from build123d import *

# Parameters (mm, degrees)
F1_DEPTH       = 1
F2_R           = 3
F4_D           = 2.75
F4_CBORE_D     = 6.2
F4_CBORE_DEPTH = 0.5
F5_W           = 40.115128
F5_H           = 5.339066
F5_W_2         = 8.616518
F5_H_2         = 40.98092
F5_W_3         = 4.081794
F5_W_4         = 16.738685
F5_H_3         = 7.16661
F5_H_4         = 1.77993
F5_W_5         = 5.194765
F5_H_5         = 9.475394
F5_H_6         = 3.222921
F6_DEPTH       = 10


with BuildPart() as f1:
    # F0 (on Top) → F1 (new body)
    with BuildSketch(Plane.XY):
        Polygon((42.5, -28), (-42.5, 28), (-42.5, -28), align=None)
        Polygon((42.5, 28), (-42.5, 28), (42.5, -28), align=None)
    extrude(amount=F1_DEPTH)

    # F2
    f2_edges = [f1.edges().sort_by_distance(p)[0] for p in [
        (-42.5, -28, 0.5),
        (-42.5, 28, 0.5),
        (42.5, -28, 0.5),
        (42.5, 28, 0.5),
    ]]
    fillet(f2_edges, radius=F2_R)

    # F4 (through all)
    with Locations(Plane.XY.offset(1)):
        with Locations((-39, 24.5), (-39, -24.5), (19, -24.5), (19, 24.5)):
            CounterBoreHole(F4_D / 2, F4_CBORE_D / 2, F4_CBORE_DEPTH)

    # F5 (on face) → F6 (join)
    with BuildSketch(Plane.XY.offset(1)):
        with Locations((-10.416318, 22.961362)):
            Rectangle(F5_W, F5_H)
        with Locations((38.191741, -0.631528)):
            Rectangle(F5_W_2, F5_H_2)
        with Locations((44.540897, -0.631528)):
            Rectangle(F5_W_3, F5_H_2)
        with Locations((-16.04398, -24.416695)):
            Rectangle(F5_W_4, F5_H_3)
        with Locations((-16.04398, -28.889965)):
            Rectangle(F5_W_4, F5_H_4)
        with Locations((8.053955, -23.262303)):
            Rectangle(F5_W_5, F5_H_5)
        with Locations((8.053955, -29.61146)):
            Rectangle(F5_W_5, F5_H_6)
    extrude(amount=F6_DEPTH)


solid = f1.part
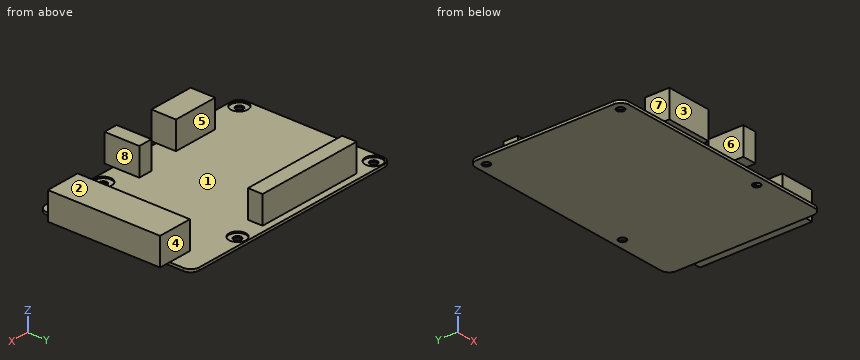
Could you check a few things on this model? Use its own coordinates, in mm. Face numbers are marked on the shaded views. A direction names the side the tool comes from. Round coordinates to 2 decimals unless told otherwise and drop trailing zeros. Write each loop counter-clockwise with the first axis right and the second up, starting at its lowest first coordinate (ties: lowest second). Pieces come first, ordered by that corner, then holes. Notation, with made-up numbers: (-10.5, 75.25) -> (32.5, 75.25) arc R17 ccw to (32.5, 87.25) -> close; hole circle Ø6 at (-35, 19.5). An arc over 180 degrees is marked (long way). Use a Markdown table: item, result.
1. If we section it at A-A (x = 19): List the corners of the cut face in (y, z) for me (3 decimals), then the cut area to 4 significant figures.
Answer key:
| item | result |
|---|---|
| outline | (-28, 0) -> (-25.875, 0) -> (-25.875, 0.5) -> (-27.6, 0.5) -> (-27.6, 1) -> (-28, 1) -> close; (-23.125, 0) -> (23.125, 0) -> (23.125, 0.5) -> (21.4, 0.5) -> (21.4, 1) -> (-21.4, 1) -> (-21.4, 0.5) -> (-23.125, 0.5) -> close; (25.875, 0) -> (28, 0) -> (28, 1) -> (27.6, 1) -> (27.6, 0.5) -> (25.875, 0.5) -> close |
| area | 47.05 mm^2 |
2. Which directions (+Z, -Z, +X, -X, +Y, -Y) give clear straight access to the entire face, cutting with the end or side of a thin tool? Please do the marked faces 4, 5, 6, 7 and 8.
Answer key:
| item | result |
|---|---|
| face 4 | +Z, +X, -X, +Y |
| face 5 | +Z, -X |
| face 6 | +Z, -Y |
| face 7 | +Z, -X, -Y |
| face 8 | +Z, +Y, -Y |
3. If we section it at B-B (z = 9.75): List the corners of the cut face in (x, y) for me.
Answer key:
| item | result |
|---|---|
| outline | (-30.47, 20.29) -> (9.64, 20.29) -> (9.64, 25.63) -> (-30.47, 25.63) -> close; (-24.41, -29.78) -> (-7.67, -29.78) -> (-7.67, -20.83) -> (-24.41, -20.83) -> close; (5.46, -31.22) -> (10.65, -31.22) -> (10.65, -18.52) -> (5.46, -18.52) -> close; (33.88, -21.12) -> (46.58, -21.12) -> (46.58, 19.86) -> (33.88, 19.86) -> close |
4. Please list where these lines run through material, in increasing order: probe 1 along Y at (x, z) = (19, 0.7); probe 2 along Y at (x, z) = (-39, 0.2) (3 decimals); probe 3 along Y at (x, z) = (-23.5, 5.5).
Answer key:
| item | result |
|---|---|
| probe 1 | y = -28 to -27.6, -21.4 to 21.4, 27.6 to 28 |
| probe 2 | y = -28 to -25.875, -23.125 to 23.125, 25.875 to 28 |
| probe 3 | y = -29.78 to -20.83, 20.29 to 25.63 |
5. We'd pull the mould along Y, two halves only. Please class the marked faces 1, 2 and 3: +Y half, -Y half, draft (parallel to the pull), parting line (faces both ways), or undercut.
Answer key:
| item | result |
|---|---|
| face 1 | undercut |
| face 2 | draft |
| face 3 | -Y half |
6. If we section it at D-D (x = 7.5): List the corners of the cut face in (y, z) for me, then the cut area to 3 significant figures.
Answer key:
| item | result |
|---|---|
| outline | (-31.22, 1) -> (-28, 1) -> (-28, 0) -> (28, 0) -> (28, 1) -> (25.63, 1) -> (25.63, 11) -> (20.29, 11) -> (20.29, 1) -> (-18.52, 1) -> (-18.52, 11) -> (-31.22, 11) -> close |
| area | 236 mm^2 |
7. For pin 1 Ø3 at (x, y) = (-20.5, 18) entering from +Z; pin 2 Ø1 at (y, z) = (10.5, 4) entering from -X; pin 3 Ø4.5 at (x, y) = (19, -24.5) entering from +Z, each with a flat end and sliding along its axis, tell me the tip position at first contact or that it passes through.
Answer key:
| item | result |
|---|---|
| pin 1 | stops at z = 1 |
| pin 2 | stops at x = 33.88 |
| pin 3 | stops at z = 0.5 |
8. If we section it at C-C (y = 17): List the corners of the cut face in (x, z) for me, then the cut area to 3 significant figures.
Answer key:
| item | result |
|---|---|
| outline | (-42.5, 0) -> (42.5, 0) -> (42.5, 1) -> (46.58, 1) -> (46.58, 11) -> (33.88, 11) -> (33.88, 1) -> (-42.5, 1) -> close |
| area | 212 mm^2 |
